```python
from build123d import *

# Parameters (mm, degrees)
SZKIC1_R                                 = 5
DODANIE_WYCI_GNI_CIE1_DEPTH              = 5
WYTNIJ_WYCI_GNI_CIE3_DEPTH               = 2.5
OTWORY_USTALAJ_CE_3_0MMCLEARANCE_1_D     = 3
OTWORY_USTALAJ_CE_3_0MMCLEARANCE_1_DEPTH = 7.25
OTWORY_USTALAJ_CE_3_0MMCLEARANCE_1_TIP   = 0.901290929
SZKIC19_W                                = 6
SZKIC19_H                                = 3.662813391
WYTNIJ_WYCI_GNI_CIE8_DEPTH               = 2.5
SZKIC20_W                                = 3
SZKIC20_H                                = 6.977009587
WYTNIJ_WYCI_GNI_CIE9_DEPTH               = 2.5


with BuildPart() as part:
    # Szkic1 → Dodanie-wyciągnięcie1 (new body)
    with BuildSketch(Plane.XY):
        Circle(SZKIC1_R)
    extrude(amount=DODANIE_WYCI_GNI_CIE1_DEPTH)

    # Szkic10 → Wytnij-wyciągnięcie3 (cut)
    with BuildSketch(Plane.XY.offset(5)):
        Polygon((0, 3.464101615), (-3, 1.732050808), (-3, -1.732050808), (0, -3.464101615), (3, -1.732050808), (3, 1.732050808), align=None)
    extrude(amount=-WYTNIJ_WYCI_GNI_CIE3_DEPTH, mode=Mode.SUBTRACT)

    # Otwory ustalające Ø3.0mmClearance 1
    with Locations(Plane.XY.offset(2.5)):
        with Locations((0, 0)):
            Hole(OTWORY_USTALAJ_CE_3_0MMCLEARANCE_1_D / 2, depth=OTWORY_USTALAJ_CE_3_0MMCLEARANCE_1_DEPTH)
            with Locations((0, 0, -(OTWORY_USTALAJ_CE_3_0MMCLEARANCE_1_DEPTH + OTWORY_USTALAJ_CE_3_0MMCLEARANCE_1_TIP / 2))):  # 118° drill point
                Cone(0, OTWORY_USTALAJ_CE_3_0MMCLEARANCE_1_D / 2, OTWORY_USTALAJ_CE_3_0MMCLEARANCE_1_TIP, mode=Mode.SUBTRACT)

    # Szkic19 → Wytnij-wyciągnięcie8 (cut)
    with BuildSketch(Plane.XY.offset(5)):
        with Locations((0, 3.563457504)):
            Rectangle(SZKIC19_W, SZKIC19_H)
    extrude(amount=-WYTNIJ_WYCI_GNI_CIE8_DEPTH, mode=Mode.SUBTRACT)

    # Szkic20 → Wytnij-wyciągnięcie9 (cut)
    with BuildSketch(Plane.XY.offset(2.5)):
        with Locations((0, 3.488504794)):
            Rectangle(SZKIC20_W, SZKIC20_H)
    extrude(amount=-WYTNIJ_WYCI_GNI_CIE9_DEPTH, mode=Mode.SUBTRACT)


solid = part.part
```
The listing builds one solid part. Answer for the finished solid, in the listing's coordinates (mm). A direction names the side the tool comes from. Coordinates: 2 decimals unless noted, no trailing zeros. Write each loop counter-clockwise with the first axis right and the second up, starting at its lowest first coordinate (ties: lowest second). Pieces come first, ordered by that corner, then holes. Notation, with made-up numbers: M 27.5,-27.5 L 83.5,-27.5 A29 cw 83.5,-3.5 Z; hole C 45,61 d11. An arc over 180 degrees is marked long. Use a Markdown table: item, result. Add a question column.
1. Which of the six approach directions +Z, -Z, +X, -X, +Y, -Y give full straight-line access (tool end or side, diameter ignored) to faces 5 (the flat face through (0, -2, 0)), 6 (the flat face through (-1.5, 2, 1)), 7 (the flat face through (1.3, -1.1, 2.5))?
2. Section A-A (y = -1.25) is taken. Give the vertices of the cut face in (x, z), plus the area to 3 significant figures.
3. Given P1, Ø2, axis at y = 1.5, z = 3.5, coming from the -X side; P2, Ø2, axis at y = 3, z = 1, coming from the +X side; P3, Ø1.5, axis at y = -3.5, z = 3.5, coming from the -X side, each flat-ended and moving along its own axis, determine where each tip first touches the part or whether it passes through.
4. Section D-D (y = 2.25) is taken. Give the vertices of the cut face in (x, z).
5. Section B-B (z = 3.5) is taken. Give the vertices of the cut face in (x, y), plus the area to 3 significant figures.
6. Section C-C (x = 4) is taken. Give the vertices of the cut face in (y, z).
7. Straight lines are drawn through the part: line 1 along X through (y, z) = (0, 4.6); line 2 along Y through (x, z) = (-4, 2.2); line 3 along Z through (x, y) = (2, 2). For each, find the intervals that lie inside material, in ascending order. Write a range as [from, to].
8. For a pull along X with two mould halves and no side action, classify faces 1 (the flat face through (-1.2, -3.4, 5)), 2 (the flat face through (3, 1, 4)), 3 (the flat face through (-3, 1, 4)), 4 (the cylindrical face through (0, -5, 2)) as +X half, -X half, draft (parallel to the pull), parting line (faces both ways), or undercut.
Data:
| question | item | result |
|---|---|---|
| 1 | face 5 | -Z, +X, -X, +Y, -Y |
| 1 | face 6 | +Z, -Z, +Y |
| 1 | face 7 | +Z, +Y |
| 2 | outline | M -4.84,0 L -0.83,0 L -0.83,2.5 L -3,2.5 L -3,5 L -4.84,5 Z; M 0.83,0 L 4.84,0 L 4.84,5 L 3,5 L 3,2.5 L 0.83,2.5 Z |
| 2 | area | 29.3 mm2 |
| 3 | P1 | stops at x = -4.97 |
| 3 | P2 | stops at x = 4.58 |
| 3 | P3 | stops at x = -4.18 |
| 4 | outline | M -4.47,0 L -1.5,0 L -1.5,2.5 L -3,2.5 L -3,5 L -4.47,5 Z; M 1.5,0 L 4.47,0 L 4.47,5 L 3,5 L 3,2.5 L 1.5,2.5 Z |
| 5 | outline | M -3,-1.73 L -3,4 A5 ccw long 3,4 L 3,-1.73 L 0,-3.46 Z |
| 5 | area | 34.9 mm2 |
| 6 | outline | M -3,0 L 3,0 L 3,5 L -3,5 Z |
| 7 | line 1 | x = [-5, -3], [3, 5] |
| 7 | line 2 | y = [-3, 3] |
| 7 | line 3 | z = [0, 2.5] |
| 8 | face 1 | draft |
| 8 | face 2 | undercut |
| 8 | face 3 | undercut |
| 8 | face 4 | parting line |
